from build123d import *

# Parameters (mm, degrees)
F0_W     = 90
F0_H     = 90
F1_DEPTH = 5
F3_D     = 5.2
F5_D     = 5.2
F6_R     = 5


with BuildPart() as f1:
    # F0 (on Front) → F1 (new body)
    with BuildSketch(Plane.XZ):
        Rectangle(F0_W, F0_H)
    extrude(amount=F1_DEPTH)

    # F3 (through all)
    with Locations(Plane.XZ.offset(5)):
        with Locations((-37.066457, 15.5), (-11.066457, 15.5), (11.066457, 15.5), (37.066457, 15.5), (37.066457, -15.5), (11.066457, -15.5), (-11.066457, -15.5), (-37.066457, -15.5)):
            Hole(F3_D / 2)

    # F5 (through all)
    with Locations(Plane.XZ.offset(5)):
        with Locations((-30, 33), (2, 33), (2, -33), (-30, -33)):
            Hole(F5_D / 2)

    # F6
    f6_edges = [f1.edges().sort_by_distance(p)[0] for p in [
        (-45, -2.5, 45),
        (-45, -2.5, -45),
        (45, -2.5, 45),
        (45, -2.5, -45),
    ]]
    fillet(f6_edges, radius=F6_R)


solid = f1.part
Work out the finished part from the listing and answer in its coordinate system (mm). Give positions to 0.01 mm unless a question says otherwise; leave off trailing zeros. Loops run counter-clockwise (first coordinate to the right, second up) from the corner with the lowest first, then second, coordinate; pieces in that order, holes last. Notation, with made-up numbers: (9.5, 73.5) -> (54.5, 73.5) arc R22 ccw to (54.5, 95.5) -> close; hole circle Ø1 at (-2.75, -18). An arc over 180 degrees is marked (long way). Use a Markdown table: item, result. Add a question column.
1) The part is cut by section C-C, the plane z = -15.5. Determine the outline of the cut face in (x, y), plus the area to 3 significant figures.
2) The part is cut by section D-D, the plane y = -3.65. Count the separate pieces of the cut face and the enclosed holes in it, plus the area to 3 significant figures.
3) For a pull along Z with two mould halves and no side action, classify faces 1 (the cylindrical face through (-9, -2.47, -17.08)), 2 (the flat face through (-1, -2, 45)), 3 (the cylindrical face through (-44, -3, -43)) as +Z half, -Z half, draft (parallel to the pull), parting line (faces both ways), or undercut.
4) Consider line 1 along Z through (x, y) = (-30, -2.15); line 2 along Z through (x, y) = (0.5, -0.45); line 3 along X through (y, z) = (-2.3, -16.5). Determine where each line is inside the solid, lowest interval first.
5) The part is cut by section B-B, the plane x = -30. Determine the outline of the cut face in (y, z).
6) The part is cut by section A-A, the plane z = -33. Determine the outline of the cut face in (x, y), plus the area to 3 significant figures.
Reported:
| question | item | result |
|---|---|---|
| 1 | outline | (-45, -5) -> (-39.67, -5) -> (-39.67, 0) -> (-45, 0) -> close; (-34.47, -5) -> (-13.67, -5) -> (-13.67, 0) -> (-34.47, 0) -> close; (-8.47, -5) -> (8.47, -5) -> (8.47, 0) -> (-8.47, 0) -> close; (13.67, -5) -> (34.47, -5) -> (34.47, 0) -> (13.67, 0) -> close; (39.67, -5) -> (45, -5) -> (45, 0) -> (39.67, 0) -> close |
| 1 | area | 346 mm^2 |
| 2 | separate pieces | 1 |
| 2 | enclosed holes | 12 |
| 2 | area | 7,820 mm^2 |
| 3 | face 1 | undercut |
| 3 | face 2 | +Z half |
| 3 | face 3 | -Z half |
| 4 | line 1 | z = -45 to -35.6, -30.4 to 30.4, 35.6 to 45 |
| 4 | line 2 | z = -45 to -35.12, -30.88 to 30.88, 35.12 to 45 |
| 4 | line 3 | x = -45 to -39.47, -34.67 to -13.47, -8.67 to 8.67, 13.47 to 34.67, 39.47 to 45 |
| 5 | outline | (-5, -45) -> (0, -45) -> (0, -35.6) -> (-5, -35.6) -> close; (-5, -30.4) -> (0, -30.4) -> (0, 30.4) -> (-5, 30.4) -> close; (-5, 35.6) -> (0, 35.6) -> (0, 45) -> (-5, 45) -> close |
| 6 | outline | (-45, -5) -> (-32.6, -5) -> (-32.6, 0) -> (-45, 0) -> close; (-27.4, -5) -> (-0.6, -5) -> (-0.6, 0) -> (-27.4, 0) -> close; (4.6, -5) -> (45, -5) -> (45, 0) -> (4.6, 0) -> close |
| 6 | area | 398 mm^2 |
